Design review of the part built by this model. Coordinates are the model's own, in mm. Give positions to 0.01 mm unless a question says otherwise; leave off trailing zeros. Loops run counter-clockwise (first coordinate to the right, second up) from the corner with the lowest first, then second, coordinate; pieces in that order, holes last. Notation, with made-up numbers: M 7,36 L 23,36 A25 ccw 23,54 Z; hole C 43.25,-19 d2. An arc over 180 degrees is marked long. Use CSV: the item, a comma, the result in double quotes.
from build123d import *

# Parameters (mm, degrees)
EXTRUDE_1_DEPTH     = 600
CUT_EXTRUDE_1_DEPTH = 600
EXTRUDE_2_DEPTH     = 100
SHELL_1_T           = -10
EXTRUDE_3_DEPTH     = 10


with BuildPart() as part:
    # Sketch 1 → Extrude 1 (new body)
    with BuildSketch(Plane(origin=(0, 0, 0), x_dir=(1, 0, 0), z_dir=(0, 1, 0))):
        with BuildLine():
            ThreePointArc((-900, 0), (-779.422863406, -450), (-450, -779.422863406))
            Line((-450, -779.422863406), (-600, -1039.230484541))
            ThreePointArc((-600, -1039.230484541), (-1039.230484541, -600), (-1200, 0))
            Line((-1200, 0), (-900, 0))
        make_face()
    extrude(amount=EXTRUDE_1_DEPTH)

    # Sketch 2 → Cut-Extrude 1 (cut)
    with BuildSketch(Plane(origin=(0, 600, 0), x_dir=(1, 0, 0), z_dir=(0, 1, 0))):
        Polygon((-57.795907874, -27.594980277), (-1097.026392415, -627.594980277), (-1080.637446236, -629.679823172), (-41.406961694, -29.679823172), align=None)
    extrude(amount=-CUT_EXTRUDE_1_DEPTH, mode=Mode.SUBTRACT)


with BuildPart() as cut_extrude_1_piece_1:
    # of the separate pieces the step leaves, piece 1, a body of its own (cut_extrude_1_pieces)
    add(part.part.solids().sort_by_distance((-600, 0, 1039.230484541))[0])



with BuildPart() as cut_extrude_1_piece_2:
    # of the separate pieces the step leaves, piece 2, a body of its own (cut_extrude_1_pieces)
    add(part.part.solids().sort_by_distance((-1200, 0, 0))[0])


with BuildPart() as cut_extrude_1_piece_1_1:
    add(cut_extrude_1_piece_1.part)

    add(cut_extrude_1_piece_2.part)  # Extrude 2 merges Cut-Extrude 1 piece 2
    # Sketch 3 → Extrude 2 (add)
    with BuildSketch(Plane.XZ):
        with BuildLine():
            Line((-825.212105372, 470.662928483), (-998.420193215, 570.664664625))
            ThreePointArc((-998.420193215, 570.664664625), (-995.929606575, 575.00022645), (-993.420193215, 579.324918663))
            Line((-993.420193215, 579.324918663), (-820.212105372, 479.323182521))
            ThreePointArc((-820.212105372, 479.323182521), (-822.723500531, 474.9996345), (-825.212105372, 470.662928483))
        make_face()
    extrude(amount=-EXTRUDE_2_DEPTH)

    # Shell 1
    shell_1_openings = [cut_extrude_1_piece_1_1.faces().sort_by_distance(p)[0] for p in [
        (-1010.404998502, 600, 268.177938118),
        (-737.451406396, 600, 740.947427754),
    ]]
    offset(amount=SHELL_1_T, openings=shell_1_openings, kind=Kind.INTERSECTION)

    # Sketch 4 → Extrude 3 (add)
    with BuildSketch(Plane(origin=(0, 600, 0), x_dir=(1, 0, 0), z_dir=(0, 1, 0))):
        with BuildLine():
            Line((-463.632780681, -783.035532194), (-603.639245264, -1025.533842239))
            ThreePointArc((-603.639245264, -1025.533842239), (-839.687348019, -843.223076995), (-1022.988355102, -607.943110271))
            Line((-1022.988355102, -607.943110271), (-780.47604659, -467.928563671))
            ThreePointArc((-780.47604659, -467.928563671), (-641.696808412, -645.232675919), (-463.632780681, -783.035532194))
        make_face()
        with BuildLine():
            Line((-909.945053286, -10), (-1189.957982451, -10))
            ThreePointArc((-1189.957982451, -10), (-1150.096279744, -305.579036124), (-1037.988355102, -581.962348158))
            Line((-1037.988355102, -581.962348158), (-795.47604659, -441.947801557))
            ThreePointArc((-795.47604659, -441.947801557), (-879.636292904, -233.109399653), (-909.945053286, -10))
        make_face()
    extrude(amount=-EXTRUDE_3_DEPTH)


solid = cut_extrude_1_piece_1_1.part
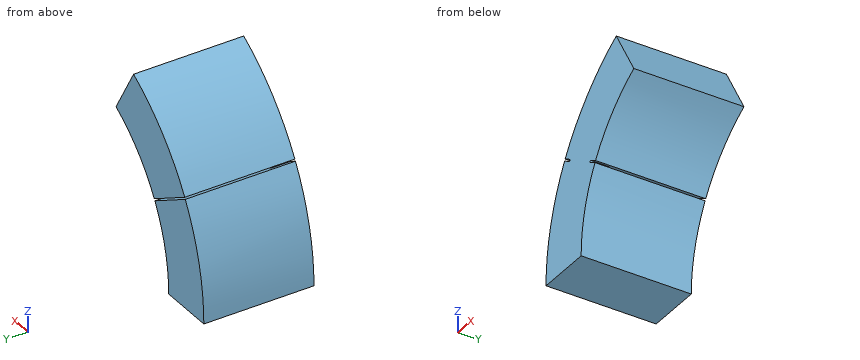
(1) Clearance check with flat-ended pins moving along their axes: P1, Ø3, axis at x = -992.5, y = 372.5, coming from the +Z side; P2, Ø1, axis at y = 477, z = 409, coming from the +X side; P3, Ø10, axis at x = -551, y = 349.5, coming from the -Z side. State where each tip first meets the part, or that it passes through.
A:
P1,"z = 676.7"
P2,"x = -801.44"
P3,"z = 707.72"
(2) We need section D-D on z = 542.5. State the section outline as (x, y) points.
A:
outline,"M -1070.37,0 L -718.12,0 L -718.12,600 L -929.64,600 L -929.64,100 L -949.64,100 L -949.64,600 L -1070.37,600 Z; hole M -1059.15,10 L -730.61,10 L -730.61,590 L -909.64,590 L -909.64,90 L -969.64,90 L -969.64,590 L -1059.15,590 Z"
(3) We need section C-C on x = -543. State the section outline as (y, z) points, then the cut area to 3 significant figures.
A:
outline,"M 0,717.74 L 600,717.74 L 600,940.5 L 0,940.5 Z; hole M 10,730.24 L 590,730.24 L 590,920.5 L 10,920.5 Z"
area,"23,300 mm²"
(4) We need section B-B on z = 679. State the section outline as (x, y) points.
A:
outline,"M -989.42,0 L -590.73,0 L -590.73,600 L -989.42,600 Z; hole M -977.27,10 L -605.85,10 L -605.85,590 L -977.27,590 Z"
(5) We need section A-A on y = 413. State the section outline as (x, z) points.
A:
outline,"M -1200,0 L -900,0 A900 cw -781.91,445.66 L -1041.72,595.66 A1200 ccw Z; M -1036.72,604.32 L -776.91,454.32 A900 cw -450,779.42 L -600,1039.23 A1200 ccw Z; hole M -1189.96,10 L -909.95,10 A910 cw -795.48,441.95 L -1037.99,581.96 A1190 ccw Z; hole M -1022.99,607.94 L -780.48,467.93 A910 cw -463.63,783.04 L -603.64,1025.53 A1190 ccw Z"
(6) Wall thickness on line 1 along Y through (x, z) = (-797, 506.5); line 2 along Z through (x, y) = (-835, 48); line 3 along Z through (x, y) = (-787, 117): over which ranges is each line inside the solid? List them lowest first. Write a range as [from, to].
A:
line 1,"[0, 10], [590, 600]"
line 2,"[335.82, 361.77], [464.77, 473.68], [847.86, 861.84]"
line 3,"[436.61, 448.6], [460.15, 471.7], [892.6, 905.89]"
